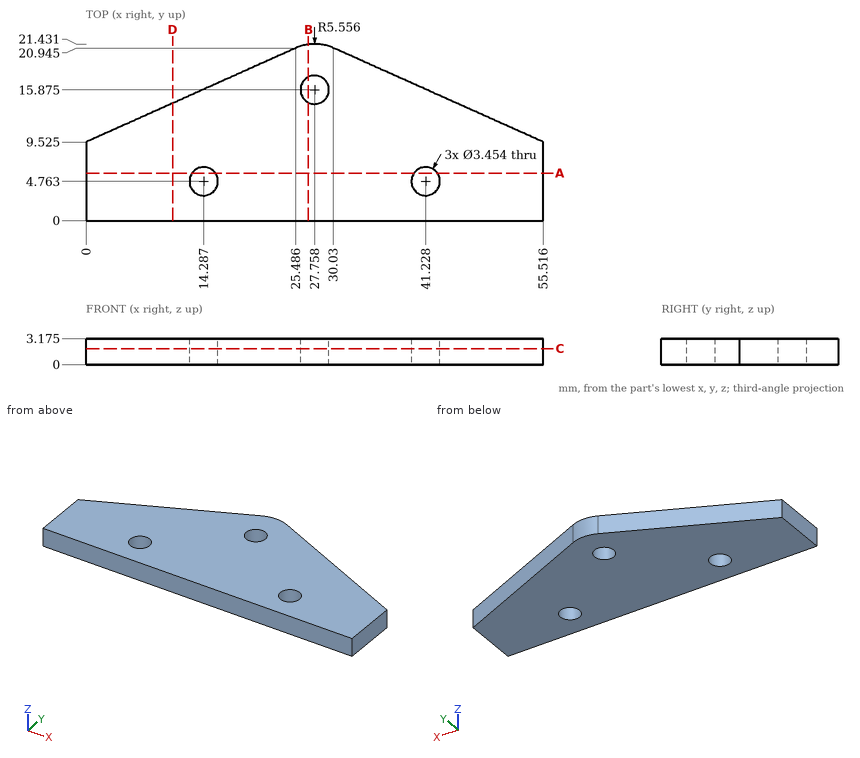
Job drawing, mm, ordinate dimensions from the low corner. One solid piece. Coordinates: 2 decimals unless noted, no trailing zeros. Loops run counter-clockwise (first coordinate to the right, second up) from the corner with the lowest first, then second, coordinate; pieces in that order, holes last. Notation, with made-up numbers: (11, 45) - (24, 45) arc R24 ccw to (24, 68) - close; hole circle Ø10 at (-2.5, -26.5). An arc over 180 degrees is marked (long way). Write item = value, one per line. Start each with the question number.
Q1. Flat gauge pins, fed straight in: pin 1 Ø1.5 at (y, z) = (11.5, 1.5) entering from -X (1 decimal); pin 2 Ø1.5 at (y, z) = (15.5, 2) entering from +X (1 decimal). Where does each tip first touch, or does it go through?
Q2. Cut at A-A, the plane y = 5.75. List the corners of the cut face in (x, z) (1 decimal), then the cut area to 3 significant figures.
Q3. Cut at D-D, the plane x = 10.5. List the corners of the cut face in (y, z) (1 decimal).
Q4. Drill centre lines: L1, parallel to Y at x = 28.5, z = 0.45 (1 decimal); L2, parallel to Y at x = 6, z = 1.6 (1 decimal); L3, parallel to X at y = 20.5, z = 1.3 (1 decimal). Where is each one in solid material? Low to high.
Q5. Cut at B-B, the plane x = 27. List the corners of the cut face in (y, z) (1 decimal).
Q6. Cut at C-C, the plane z = 1.95. List the corners of the cut face in (x, y) (1 decimal), then the cut area to 3 significant figures.
Computed:
q1.pin_1 = 2.7
q1.pin_2 = 43.9
q2.outline = (0, 0) - (12.9, 0) - (12.9, 3.2) - (0, 3.2) - close; (15.7, 0) - (39.8, 0) - (39.8, 3.2) - (15.7, 3.2) - close; (42.6, 0) - (55.5, 0) - (55.5, 3.2) - (42.6, 3.2) - close
q2.area = 158 mm²
q3.outline = (0, 0) - (14.2, 0) - (14.2, 3.2) - (0, 3.2) - close
q4.L1 = 0 to 14.3, 17.4 to 21.4
q4.L2 = 0 to 12.2
q4.L3 = 24.5 to 31
q5.outline = (0, 0) - (14.3, 0) - (14.3, 3.2) - (0, 3.2) - close; (17.4, 0) - (21.4, 0) - (21.4, 3.2) - (17.4, 3.2) - close
q6.outline = (0, 0) - (55.5, 0) - (55.5, 9.5) - (30, 20.9) arc R5.6 ccw to (25.5, 20.9) - (0, 9.5) - close; hole circle Ø3.5 at (14.3, 4.8); hole circle Ø3.5 at (27.8, 15.9); hole circle Ø3.5 at (41.2, 4.8)
q6.area = 845 mm²
